```python
from build123d import *

# Parameters (mm, degrees)
SKETCH3_R          = 2.5
SKETCH7_W          = 6.517782954
SKETCH7_H          = 4.322109435
CUT_EXTRUDE1_DEPTH = 72


with BuildPart() as part:
    # Sweep1: sweep along a path in Sketch4
    with BuildLine(Plane.XY) as sweep1_path:
        Line((0, 0), (0, 130))
        ThreePointArc((0, 130), (2.928932188, 137.071067812), (10, 140))
        Line((10, 140), (50, 140))
        ThreePointArc((50, 140), (57.071067812, 137.071067812), (60, 130))
        Line((60, 130), (60, 24.600902506))
        Line((60, 24.600902506), (60, 0))
    # Sketch3 → Sweep1 (sweep)
    with BuildSketch(Plane(origin=(0, 0, 0), x_dir=(1, 0, 0), z_dir=(0, 1, 0))):
        Circle(SKETCH3_R)
    sweep(path=sweep1_path.line)

    # Sketch5 → Revolve1 (revolve)
    with BuildSketch(Plane.XY):
        with BuildLine():
            Line((0, 0), (0, -4.2))
            add(Edge.make_bspline(
                [(0.921927602, -3.641780971), (0.629243953, -4.327906562), (0, -4.2)],
                knots=[0, 0, 0, 1, 1, 1], degree=2))
            Line((0.921927602, -3.641780971), (2.5, 0))
            Line((2.5, 0), (0, 0))
        make_face()
    revolve(axis=Axis((0, 0, 0), (0, -1, 0)))

    # Sketch6 → Revolve2 (revolve)
    with BuildSketch(Plane.XY):
        with BuildLine():
            Line((57.5, 0), (60, 0))
            Line((60, 0), (60, -4))
            add(Edge.make_bspline(
                [(59.123790654, -3.437958358), (59.375682143, -4.137387225), (60, -4)],
                knots=[0, 0, 0, 1, 1, 1], degree=2))
            Line((59.123790654, -3.437958358), (57.5, 0))
        make_face()
    revolve(axis=Axis((60, 0, 0), (0, -1, 0)))

    # Sketch7 → Cut-Extrude1 (cut)
    with BuildSketch(Plane(origin=(0, 0, 0), x_dir=(0, 0, -1), z_dir=(1, 0, 0))):
        with Locations((-0.143512102, 142.161054718)):
            Rectangle(SKETCH7_W, SKETCH7_H)
    extrude(amount=CUT_EXTRUDE1_DEPTH, mode=Mode.SUBTRACT)


solid = part.part
```
Part model, mm, in its own coordinate system. Round coordinates to 2 decimals unless told otherwise and drop trailing zeros. Order: outer loops, then holes, each group sorted by start corner. A loop starts at its lowest first (then second) coordinate and runs counter-clockwise, first axis right, second up. Notation, with made-up numbers: M 87,32 L 142,32 A18 cw 142,56 Z; hole C 55.25,79.25 d1. An arc over 180 degrees is marked long. Put each result on its own line as item: value. Start each with the question number.
1. Slice it at B-B on x = 36. List the corners of the cut face in (y, z), then the cut area to 3 significant figures.
2. Two-plate mould, pull along X, no slides. Class faces 1 (the face through (58.723, -2.459, -0.402)), 2 (the face through (30, 140, 0)), 3 (the face through (57.69, 64.09, 0.96)): +X half, -X half, draft (parallel to the pull), parting line (faces both ways), or undercut.
3. Slice it at A-A on y = 44. List the corners of the cut face in (x, z).
4. Drill centre lines: probe 1 along X at (y, z) = (69.5, -0.25); probe 2 along Y at (x, z) = (29, -0.25); probe 3 along X at (y, z) = (113, 1.5). Where is each one in solid material? Low to high. Write a range as [from, to].
Findings:
1. outline: M 140,-2.5 L 140,2.5 A2.5 ccw Z
1. area: 9.82 mm2
2. face 1: undercut
2. face 2: draft
2. face 3: undercut
3. outline: C 0,0 d5; C 60,0 d5
4. probe 1: [-2.49, 2.49], [57.51, 62.49]
4. probe 2: [137.51, 140]
4. probe 3: [-2, 2], [58, 62]
